Job drawing, mm, ordinate dimensions from the low corner. One solid piece. Give positions to 0.01 mm unless a question says otherwise; leave off trailing zeros. Loops run counter-clockwise (first coordinate to the right, second up) from the corner with the lowest first, then second, coordinate; pieces in that order, holes last. Notation, with made-up numbers: (51.5, 71.5) - (86.5, 71.5) arc R15 cw to (86.5, 79.5) - close; hole circle Ø2 at (39, 60.5). An arc over 180 degrees is marked (long way). Use a Markdown table: item, result.
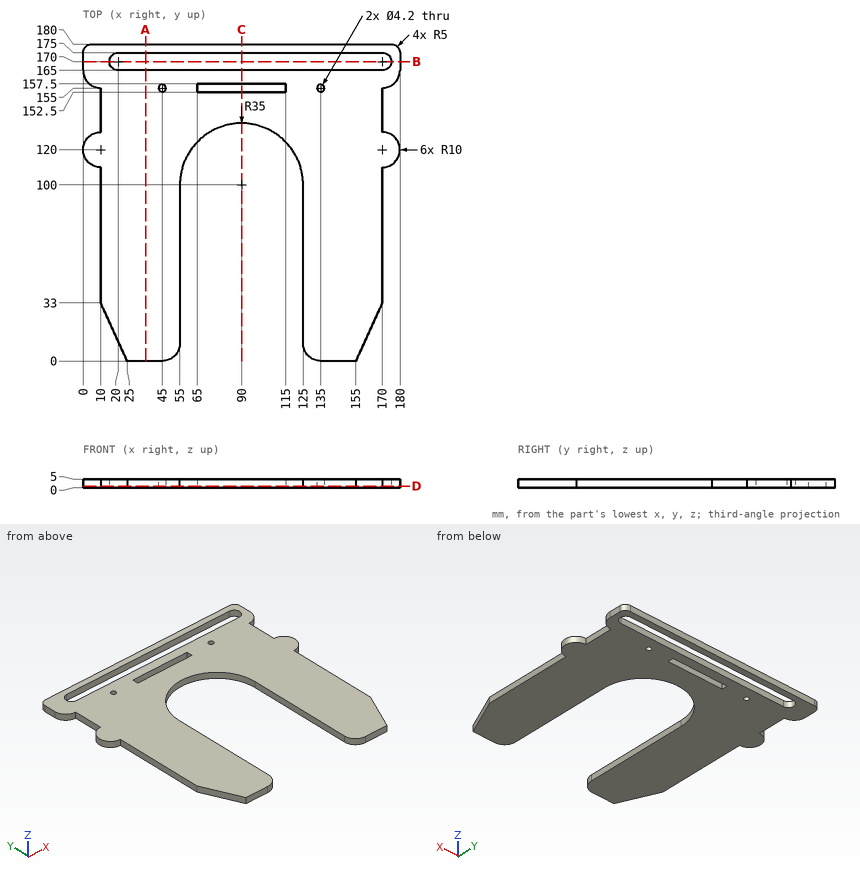
(1) Slice it at C-C, the plane x = 90. Write the cut outline in (y, z).
Computed:
| item | result |
|---|---|
| outline | (135, 0) - (152.5, 0) - (152.5, 5) - (135, 5) - close; (157.5, 0) - (165, 0) - (165, 5) - (157.5, 5) - close; (175, 0) - (180, 0) - (180, 5) - (175, 5) - close |
(2) Drill centre lines: probe 1 along Y at (x, z) = (45, 3.35); probe 2 along Y at (x, z) = (40, 4.45); probe 3 along X at (y, z) = (61.5, 2.5). Where is each one in solid material? Low to high. Write a range as [from, to].
Computed:
| item | result |
|---|---|
| probe 1 | [0, 152.9], [157.1, 165], [175, 180] |
| probe 2 | [0, 165], [175, 180] |
| probe 3 | [10, 55], [125, 170] |
(3) Slice it at A-A, the plane x = 35.5. Write the cut outline in (y, z), plus the area to 3 significant figures.
Computed:
| item | result |
|---|---|
| outline | (0, 0) - (165, 0) - (165, 5) - (0, 5) - close; (175, 0) - (180, 0) - (180, 5) - (175, 5) - close |
| area | 850 mm² |
(4) Slice it at D-D, the plane z = 1. Count the separate pieces of the cut face and the enclosed holes in it, plus the area to 3 significant figures.
Computed:
| item | result |
|---|---|
| separate pieces | 1 |
| enclosed holes | 4 |
| area | 18,200 mm² |
(5) Slice it at B-B, the plane y = 170. Write the cut outline in (x, z).
Computed:
| item | result |
|---|---|
| outline | (0, 0) - (15, 0) - (15, 5) - (0, 5) - close; (175, 0) - (180, 0) - (180, 5) - (175, 5) - close |
(6) Pin check, flat tips, straight feed: P1, Ø3, axis at x = 92.5, z = 2.5, coming from the -Y side; P2, Ø2.5, axis at x = 135, y = 155, coming from the -Z side; P3, Ø1.5, axis at x = 103, z = 3.5, coming from the -Y side; P4, Ø2.5, axis at x = 96, z = 2, coming from the -Y side. Stop position of each tip, or through.
Computed:
| item | result |
|---|---|
| P1 | y = 134.77 |
| P2 | through |
| P3 | y = 132.19 |
| P4 | y = 134.24 |
